Geometry: see drawing. Coordinates: mm, zero at the bounding-box minimum. Give positions to 0.01 mm unless a question says otherwise; leave off trailing zeros. Loops run counter-clockwise (first coordinate to the right, second up) from the corner with the lowest first, then second, coordinate; pieces in that order, holes last. Notation, with made-up numbers: (8.5, -1) - (35.5, -1) arc R13 cw to (35.5, 17) - close; hole circle Ø2 at (51.5, 42). An arc over 180 degrees is marked (long way). Use one line per item in the form item = value.
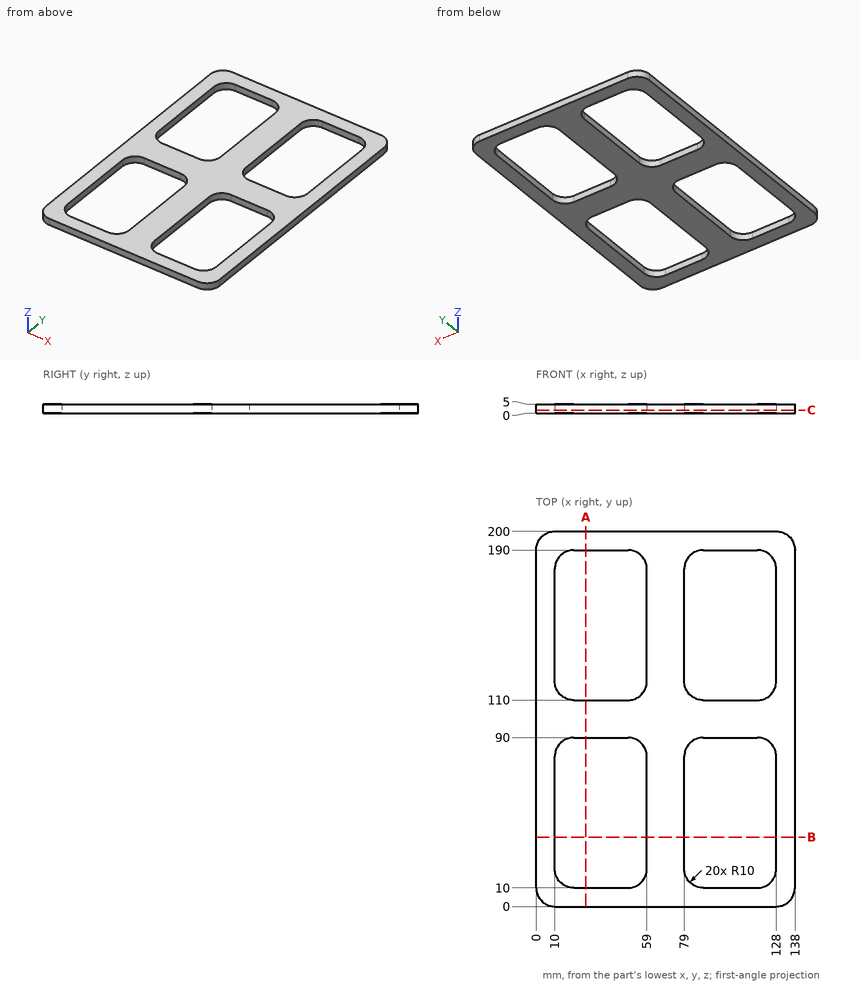
(1) Cut plane A-A (x = 26.5). Return the cut outline in (y, z).
Solution:
outline = (0, 0) - (10, 0) - (10, 5) - (0, 5) - close; (90, 0) - (110, 0) - (110, 5) - (90, 5) - close; (190, 0) - (200, 0) - (200, 5) - (190, 5) - close
(2) Cut plane B-B (y = 37). Return the cut outline in (x, z), plus the area to 3 significant figures.
Solution:
outline = (0, 0) - (10, 0) - (10, 5) - (0, 5) - close; (59, 0) - (79, 0) - (79, 5) - (59, 5) - close; (128, 0) - (138, 0) - (138, 5) - (128, 5) - close
area = 200 mm2
(3) Pin query (flat end, axial travel): P1, Ø10, axis at x = 16, y = 57.5, coming from the +Z side (1 decimal). Return the tip coordinate at first contact, or that it passes through.
Solution:
P1 = through
(4) Cut plane C-C (z = 1.8). Give the number of separate pieces and of enclosed holes in the cut face, plus the area to 3 significant figures.
Solution:
separate_pieces = 1
enclosed_holes = 4
area = 12,200 mm2
(5) Material intervals for L1, parallel to X at y = 78.5, z = 1.45; L2, parallel to Y at x = 48.5, z = 0.8; L3, parallel to Y at x = 122, z = 1.3, sorted ascending. Write a range as from..to.
Solution:
L1 = 0..10, 59..79, 128..138
L2 = 0..10, 90..110, 190..200
L3 = 0..10.83, 89.17..110.83, 189.17..200
